Read the model definition and answer for the solid it produces. Units are mm, in the model's axes. Coordinates: 2 decimals unless noted, no trailing zeros. Write each loop counter-clockwise with the first axis right and the second up, starting at its lowest first coordinate (ties: lowest second). Pieces come first, ordered by that corner, then holes.
1) Determine the mould class of faces 1 (the face through (116, 31, 0)), 2 (the face through (44.1, 15.86, 0.79)), 3 (the face through (4.75, 4.15, 0.81)), 4 (the face through (49.75, 58.95, 0.81)) for opening direction Y: +Y half, -Y half, draft (parallel to the pull), parting line (faces both ways), or undercut.
2) Find the intervals of material crossed by line 1 (Y direction, x = 177.9, z = 0.9); line 2 (Y direction, x = 178, z = 1); line 3 (X direction, y = 59, z = 0.4), in increasing order.
3) The part is cut by section A-A (x = 168). Determine the outline of the cut face in (y, z).
4) The part is cut by section C-C (x = 94). Determine the outline of the cut face in (y, z).
5) The part is cut by section D-D (y = 34.5). Determine the outline of the cut face in (x, z).
6) Each of these flat-tipped pins is pushed along its axis until it touches: pin 1 Ø4 at (x, y) = (6, 3) entering from +Z; pin 2 Ø0.5 at (y, z) = (46, 0.5) entering from +X; pin 3 Ø0.5 at (y, z) = (38, 0.5) entering from -X; pin 4 Ø0.7 at (y, z) = (-2.5, 0.5) entering from +X. Where does it stop, or does it pass through?
7) The part is cut by section B-B (y = 57.8). Determine the outline of the cut face in (x, z), then the cut area to 3 significant figures.
from build123d import *

# Parameters (mm, degrees)
BOSS_EXTRUDE1_DEPTH  = 1.6
SKETCH4_R            = 0.6
SKETCH4_R_2          = 0.8
CUT_EXTRUDE1_DEPTH   = 2.6
CUT_EXTRUDE2_DEPTH   = 2.6
CUT_EXTRUDE3_DEPTH   = 2.6
FILLET1_R            = 0.4
M3_CLEARANCE_HOLE1_D = 3.4


with BuildPart() as part:
    # Sketch2 → Boss-Extrude1 (new body)
    with BuildSketch(Plane.XY):
        with BuildLine():
            Line((68, -2), (68, -3))
            Line((68, -3), (0, -3))
            Line((0, -3), (0, 0))
            Line((0, 0), (0, 15))
            Line((0, 15), (42, 15))
            ThreePointArc((42, 15), (44.121320344, 15.878679656), (45, 18))
            Line((45, 18), (45, 63.8))
            Line((45, 63.8), (188, 63.8))
            Line((188, 63.8), (188, 0))
            Line((188, 0), (70, 0))
            ThreePointArc((70, 0), (68.585786438, -0.585786438), (68, -2))
        make_face()
    extrude(amount=BOSS_EXTRUDE1_DEPTH)

    # Sketch4 → Cut-Extrude1 (cut, through all)
    with BuildSketch(Plane(origin=(0, 0, 0), x_dir=(-1, 0, 0), z_dir=(0, 0, -1))):
        with Locations((-177.9, 46.591)):
            Circle(SKETCH4_R)
        with Locations((-177.9, 7.651)):
            Circle(SKETCH4_R_2)
        with BuildLine():
            Line((-188, 49.271), (-188, 48.871))
            Line((-188, 48.871), (-188, 5.371))
            Line((-188, 5.371), (-188, 4.971))
            ThreePointArc((-188, 4.971), (-187.882842712, 5.253842712), (-187.6, 5.371))
            Line((-187.6, 5.371), (-181.1, 5.371))
            ThreePointArc((-181.1, 5.371), (-180.817157288, 5.488157288), (-180.7, 5.771))
            Line((-180.7, 5.771), (-180.7, 9.721))
            ThreePointArc((-180.7, 9.721), (-180.817157288, 10.003842712), (-181.1, 10.121))
            Line((-181.1, 10.121), (-181.3, 10.121))
            ThreePointArc((-181.3, 10.121), (-181.582842712, 10.238157288), (-181.7, 10.521))
            Line((-181.7, 10.521), (-181.7, 43.721))
            ThreePointArc((-181.7, 43.721), (-181.582842712, 44.003842712), (-181.3, 44.121))
            Line((-181.3, 44.121), (-181.1, 44.121))
            ThreePointArc((-181.1, 44.121), (-180.817157288, 44.238157288), (-180.7, 44.521))
            Line((-180.7, 44.521), (-180.7, 48.471))
            ThreePointArc((-180.7, 48.471), (-180.817157288, 48.753842712), (-181.1, 48.871))
            Line((-181.1, 48.871), (-187.6, 48.871))
            ThreePointArc((-187.6, 48.871), (-187.882842712, 48.988157288), (-188, 49.271))
        make_face()
    extrude(amount=-CUT_EXTRUDE1_DEPTH, mode=Mode.SUBTRACT)

    # Sketch5 → Cut-Extrude2 (cut, through all)
    with BuildSketch(Plane.XY.offset(1.6)):
        with BuildLine():
            Line((15.75, 15), (17.25, 15))
            Line((17.25, 15), (17.25, 10))
            ThreePointArc((17.25, 10), (16.5, 9.25), (15.75, 10))
            Line((15.75, 10), (15.75, 15))
        make_face()
    extrude(amount=-CUT_EXTRUDE2_DEPTH, mode=Mode.SUBTRACT)

    # Sketch6 → Cut-Extrude3 (cut, through all)
    with BuildSketch(Plane.XY.offset(1.6)):
        with BuildLine():
            Line((188, 63.8), (184, 63.8))
            Line((184, 63.8), (184, 54.271))
            ThreePointArc((184, 54.271), (184.117157288, 53.988157288), (184.4, 53.871))
            Line((184.4, 53.871), (187.6, 53.871))
            ThreePointArc((187.6, 53.871), (187.882842712, 53.753842712), (188, 53.471))
            Line((188, 53.471), (188, 53.871))
            Line((188, 53.871), (188, 63.8))
        make_face()
    extrude(amount=-CUT_EXTRUDE3_DEPTH, mode=Mode.SUBTRACT)

    # Fillet1
    fillet1_edges = [part.edges().sort_by_distance(p)[0] for p in [
        (15.75, 15, 0.8),
        (17.25, 15, 0.8),
        (184, 63.8, 0.8),
        (0, 15, 0.8),
        (45, 63.8, 0.8),
        (188, 0, 0.8),
        (68, -3, 0.8),
        (0, -3, 0.8),
    ]]
    fillet(fillet1_edges, radius=FILLET1_R)

    # M3 Clearance Hole1 (through all)
    with Locations(Plane(origin=(0, 0, 0), x_dir=(-1, 0, 0), z_dir=(0, 0, -1))):
        with Locations((-178, 57.8), (-51, 57.8), (-6, 3), (-168, 6), (-51, 43.8)):
            Hole(M3_CLEARANCE_HOLE1_D / 2)


solid = part.part
Reported:
1. face 1: draft
1. face 2: +Y half
1. face 3: undercut
1. face 4: undercut
2. line 1: y = 0 to 6.85, 8.45 to 45.99, 47.19 to 56.1, 59.5 to 63.8
2. line 2: y = 0 to 6.86, 8.44 to 46, 47.18 to 56.1, 59.5 to 63.8
2. line 3: x = 45 to 49.8, 52.2 to 176.8, 179.2 to 184
3. outline: (0, 0) - (4.3, 0) - (4.3, 1.6) - (0, 1.6) - close; (7.7, 0) - (63.8, 0) - (63.8, 1.6) - (7.7, 1.6) - close
4. outline: (0, 0) - (63.8, 0) - (63.8, 1.6) - (0, 1.6) - close
5. outline: (45, 0) - (181.7, 0) - (181.7, 1.6) - (45, 1.6) - close
6. pin 1: stops at z = 1.6
6. pin 2: stops at x = 180.7
6. pin 3: stops at x = 45
6. pin 4: stops at x = 68
7. outline: (45, 0) - (49.3, 0) - (49.3, 1.6) - (45, 1.6) - close; (52.7, 0) - (176.3, 0) - (176.3, 1.6) - (52.7, 1.6) - close; (179.7, 0) - (184, 0) - (184, 1.6) - (179.7, 1.6) - close
7. area: 212 mm2
